For this review, use the dimensioned drawing (mm, ordinates from the lowest corner) and the shaded views. A direction names the side the tool comes from. Coordinates: 2 decimals unless noted, no trailing zeros. Write each loop counter-clockwise with the first axis right and the second up, starting at its lowest first coordinate (ties: lowest second). Pieces come first, ordered by that corner, then holes. Notation, with made-up numbers: M -5.75,38.25 L 17.25,38.25 A23 cw 17.25,57.25 Z; hole C 32,71.5 d3. An arc over 180 degrees is marked long. Return JSON: item names as keys, results as strings.
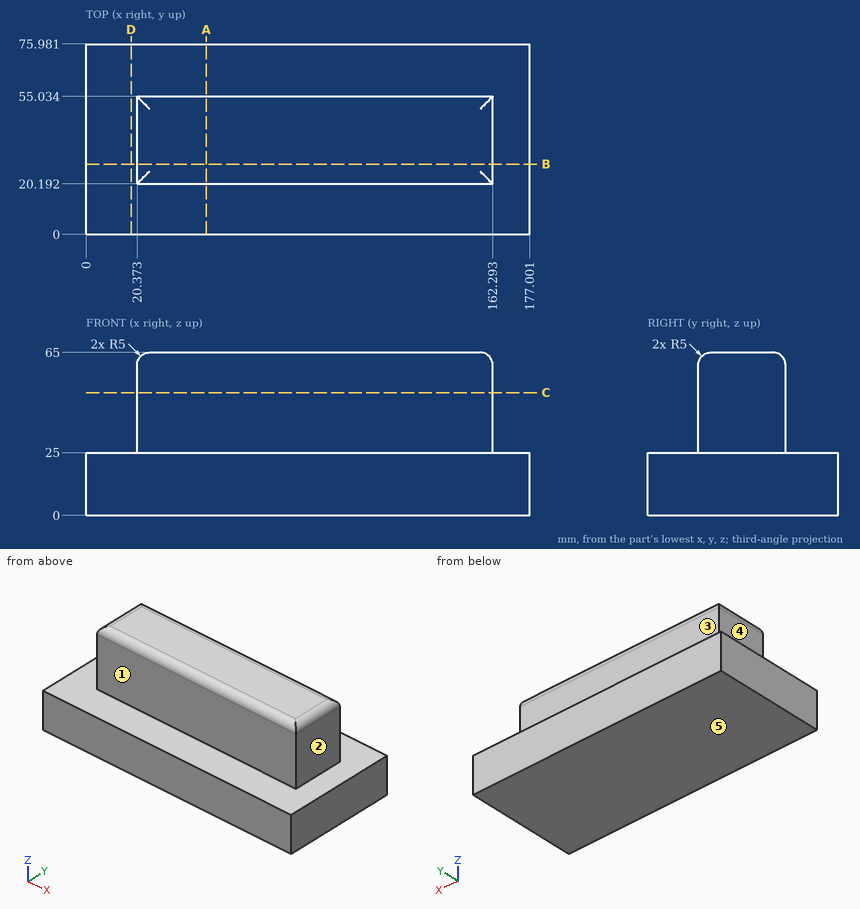
1. We need section C-C (z = 49). State the section outline as (x, y) points (1 decimal).
Checks:
{"outline": "M 20.4,20.2 L 162.3,20.2 L 162.3,55 L 20.4,55 Z"}
2. For the marked faces 1, 2, 3, 4 and 5, list the 3-axis set-ups (+Z, -Z, +X, -X, +Y, -Y) from which the entire face can be reached by the end or side of a thin tool; tool diameter is ignored.
Checks:
{"face 1": "+Z, +X, -X, -Y", "face 2": "+Z, +X, +Y, -Y", "face 3": "+Z, +X, -X, +Y", "face 4": "+Z, -X, +Y, -Y", "face 5": "-Z, +X, -X, +Y, -Y"}
3. We need section D-D (x = 18). State the section outline as (y, z) points.
Checks:
{"outline": "M 0,0 L 75.98,0 L 75.98,25 L 0,25 Z"}
4. We need section A-A (x = 48). State the section outline as (y, z) points (1 decimal), plus the area to 3 significant figures.
Checks:
{"outline": "M 0,0 L 76,0 L 76,25 L 55,25 L 55,60 A5 ccw 50,65 L 25.2,65 A5 ccw 20.2,60 L 20.2,25 L 0,25 Z", "area": "3,280 mm2"}
5. Clearance check with flat-ended pins moving along their axes: pin 1 Ø6 at (x, z) = (98, 38.5) entering from -Y; pin 2 Ø17.5 at (y, z) = (35.5, 43) entering from -X; pin 3 Ø10.5 at (y, z) = (33.5, 34.5) entering from +X. State where each tip first meets the part, or that it passes through.
Checks:
{"pin 1": "y = 20.19", "pin 2": "x = 20.37", "pin 3": "x = 162.29"}
6. Wall thickness on L1, parallel to Y at x = 21, z = 42 (1 decimal); L2, parallel to Z at x = 86, y = 25; L3, parallel to X at y = 44.5, z = 34.5: over which ranges is each line inside the solid? List them lowest first. Write a range as from..to.
Checks:
{"L1": "20.2..55", "L2": "0..65", "L3": "20.37..162.29"}
7. We need section B-B (y = 28). State the section outline as (x, z) points, plus the area to 3 significant figures.
Checks:
{"outline": "M 0,0 L 177,0 L 177,25 L 162.29,25 L 162.29,60 A5 ccw 157.29,65 L 25.37,65 A5 ccw 20.37,60 L 20.37,25 L 0,25 Z", "area": "10,100 mm2"}
